Build history of the part. All positions in model axes, mm. A direction names the side the tool comes from. Give positions to 0.01 mm unless a question says otherwise; leave off trailing zeros. Order: outer loops, then holes, each group sorted by start corner. A loop starts at its lowest first (then second) coordinate and runs counter-clockwise, first axis right, second up. Notation, with made-up numbers: (11, 60) - (43, 60) arc R24 cw to (43, 91) - close; hole circle Ø8 at (-3.75, 46.5). An arc over 180 degrees is marked (long way). Answer in a Markdown table with one row per item.
```python
from build123d import *

# Parameters (mm, degrees)
F1_DEPTH = 26


with BuildPart() as f1:
    # F0 (on Front) → F1 (new body)
    with BuildSketch(Plane.XZ):
        with BuildLine():
            ThreePointArc((522.115478, -370), (526.65902, -367.087157), (525.908713, -361.74249))
            Line((525.908713, -361.74249), (245.312642, -35))
            ThreePointArc((245.312642, -35), (243.49537, -22.055015), (254.5, -15))
            Line((254.5, -15), (274.5, -15))
            Line((274.5, -15), (274.5, 0))
            Line((274.5, 0), (30, 0))
            Line((30, 0), (30, -45))
            Line((30, -45), (-30, -45))
            Line((-30, -45), (-30, 0))
            Line((-30, 0), (-274.5, 0))
            Line((-274.5, 0), (-274.5, -15))
            Line((-274.5, -15), (-254.5, -15))
            ThreePointArc((-254.5, -15), (-243.49537, -22.055015), (-245.312642, -35))
            Line((-245.312642, -35), (-525.908713, -361.74249))
            ThreePointArc((-525.908713, -361.74249), (-526.65902, -367.087157), (-522.115478, -370))
            Line((-522.115478, -370), (-500.930536, -370))
            ThreePointArc((-500.930536, -370), (-494.044191, -368.777067), (-488, -365.257826))
            Line((-488, -365.257826), (-175, -100))
            ThreePointArc((-175, -100), (-103.279947, -82.867809), (-30, -74.662483))
            ThreePointArc((-30, -74.662483), (0, -73.912014), (30, -74.662483))
            ThreePointArc((30, -74.662483), (103.279947, -82.867809), (175, -100))
            Line((175, -100), (488, -365.257826))
            ThreePointArc((488, -365.257826), (494.044191, -368.777067), (500.930536, -370))
            Line((500.930536, -370), (522.115478, -370))
        make_face()
    extrude(amount=F1_DEPTH)


solid = f1.part
```
1. Which spindle directions (+Z, -Z, +X, -X, +Y, -Y) get a long thin tool onto all of the face, cutting with end or side? Do faces 1 (the face through (0, -13, -45)), 2 (the face through (-265, -13, -15)), 3 (the face through (-333.691, -12.818, -234.486)). Say none if no direction does.
Check result:
| item | result |
|---|---|
| face 1 | +Z, +Y, -Y |
| face 2 | -X, +Y, -Y |
| face 3 | -Z, +Y, -Y |
2. Probe line 1 (X direction, y = -15, z = -211.5); line 2 (X direction, y = -22, z = -242); line 3 (Z direction, x = 482.5, y = -14). List the from-to ranges inside material, lowest first.
Check result:
| item | result |
|---|---|
| line 1 | x = -396.89 to -306.57, 306.57 to 396.89 |
| line 2 | x = -423.08 to -342.56, 342.56 to 423.08 |
| line 3 | z = -360.6 to -311.19 |
3. Drop flat-ended pins along their axis: P1, Ø10, axis at x = 263.5, y = -9, coming from the -Z side; P2, Ø2, axis at y = -21.5, z = -295.5, coming from the -X side; P3, Ø8, axis at y = -7.5, z = -31, coming from the +X side. Give the stop position or say it passes through.
Check result:
| item | result |
|---|---|
| P1 | stops at z = -179.24 |
| P2 | stops at x = -469.88 |
| P3 | stops at x = 245.31 |
4. Cut at B-B on z = -209. Write the cut outline in (x, y).
Check result:
| item | result |
|---|---|
| outline | (-394.74, -26) - (-303.62, -26) - (-303.62, 0) - (-394.74, 0) - close; (303.62, -26) - (394.74, -26) - (394.74, 0) - (303.62, 0) - close |
5. Cut at C-C on z = -166.5. Write the cut outline in (x, y).
Check result:
| item | result |
|---|---|
| outline | (-358.24, -26) - (-253.47, -26) - (-253.47, 0) - (-358.24, 0) - close; (253.47, -26) - (358.24, -26) - (358.24, 0) - (253.47, 0) - close |
6. Cut at A-A on y = -18.5. Write the cut outline in (x, z), and give its area (3 significant figures).
Check result:
| item | result |
|---|---|
| outline | (-525.91, -361.74) arc R5 ccw to (-522.12, -370) - (-500.93, -370) arc R20 ccw to (-488, -365.26) - (-175, -100) arc R600 cw to (-30, -74.66) arc R600 cw to (30, -74.66) arc R600 cw to (175, -100) - (488, -365.26) arc R20 ccw to (500.93, -370) - (522.12, -370) arc R5 ccw to (525.91, -361.74) - (245.31, -35) arc R12.11 cw to (254.5, -15) - (274.5, -15) - (274.5, 0) - (30, 0) - (30, -45) - (-30, -45) - (-30, 0) - (-274.5, 0) - (-274.5, -15) - (-254.5, -15) arc R12.11 cw to (-245.31, -35) - close |
| area | 89,300 mm² |
7. Two-plate mould, pull along X, no slides. Class faces 4 (the face through (-30, -13, -23)), 5 (the face through (102.26, -12.82, -82.69)), 6 (the face through (243.416, -12.818, -22.231)), 7 (the face through (-512, -13, -370)): +X half, -X half, draft (parallel to the pull), parting line (faces both ways), or undercut.
Check result:
| item | result |
|---|---|
| face 4 | undercut |
| face 5 | undercut |
| face 6 | +X half |
| face 7 | draft |
8. Cut at D-D on x = -188.5. Write the cut outline in (y, z), and give its area (3 significant figures).
Check result:
| item | result |
|---|---|
| outline | (-26, -111.44) - (0, -111.44) - (0, 0) - (-26, 0) - close |
| area | 2,900 mm² |
